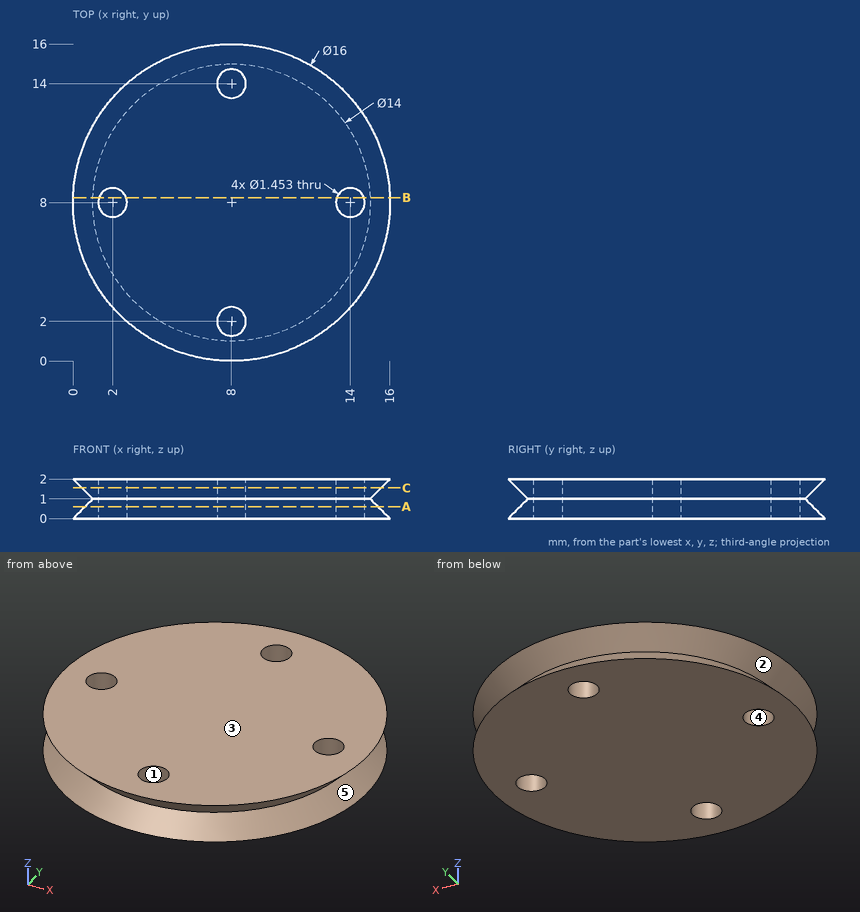
Here's the drawing with two shaded views (mm, measured from the low corner). I have some questions. A direction names the side the tool comes from. Give positions to 0.01 mm unless a question says otherwise; leave off trailing zeros. Order: outer loops, then holes, each group sorted by start corner. A loop starts at its lowest first (then second) coordinate and runs counter-clockwise, first axis right, second up. Notation, with made-up numbers: (-8.5, 8) -> (46.5, 8) arc R26 ccw to (46.5, 30) -> close; hole circle Ø8 at (76.25, 71.5). An arc over 180 degrees is marked (long way). Use a Markdown table: item, result. Add a question column.
Item 1: Imagine slicing it at B-B on y = 8.25. Give the number of separate pieces and of enclosed holes in the cut face, plus the area to 3 significant figures.
Item 2: Imagine slicing it at C-C on z = 1.55. Please give me the cut outline in (x, y).
Item 3: I need wall thicknesses on line 1 (Z direction, x = 10.5, y = 1); line 2 (Y direction, x = 2.25, z = 1.65) (1 decimal); line 3 (Y direction, x = 14, z = 0.9) (1 decimal). Which ranges of each line are inside material? Lowest first, please.
Item 4: If we mould it in two halves opening along X, with no side actions, what happens to the marked faces 1, 2 and 3? For each: pulls with the +X half, pulls with the -X half, needs draft (parallel to the pull), parting line crosses it, or undercut.
Item 5: Imagine slicing it at A-A on z = 0.6. Please give me the cut outline in (x, y).
Item 6: For the marked faces 4 and 5, which set-ups out of +Z, -Z, +X, -X, +Y, -Y let a thin tool reach every point of the face, with its end or its side?
Item 7: Will this pin go through, and if not, where does the flat tip stop? pin 1 (0.9 mm diameter, centred on x = 8, y = 2, fed in from -Z).
Data:
| question | item | result |
|---|---|---|
| 1 | separate pieces | 3 |
| 1 | enclosed holes | 0 |
| 1 | area | 24.5 mm² |
| 2 | outline | circle Ø15.1 at (8, 8); hole circle Ø1.45 at (2, 8); hole circle Ø1.45 at (8, 2); hole circle Ø1.45 at (8, 14); hole circle Ø1.45 at (14, 8) |
| 3 | line 1 | z = 0 to 0.57, 1.43 to 2 |
| 3 | line 2 | y = 3 to 7.3, 8.7 to 13 |
| 3 | line 3 | y = 4.2 to 7.3, 8.7 to 11.8 |
| 4 | face 1 | undercut |
| 4 | face 2 | parting line crosses it |
| 4 | face 3 | needs draft |
| 5 | outline | circle Ø14.8 at (8, 8); hole circle Ø1.45 at (2, 8); hole circle Ø1.45 at (8, 2); hole circle Ø1.45 at (8, 14); hole circle Ø1.45 at (14, 8) |
| 6 | face 4 | +Z, -Z |
| 6 | face 5 | none |
| 7 | pin 1 | passes through |
